Could you check a few things on this drawing? It's one solid part, dimensions in mm from its lowest x, y, z. A direction names the side the tool comes from. Coordinates: 2 decimals unless noted, no trailing zeros. Loops run counter-clockwise (first coordinate to the right, second up) from the corner with the lowest first, then second, coordinate; pieces in that order, holes last. Notation, with made-up numbers: M -37.5,20.25 L -1.5,20.25 A24 ccw -1.5,32.25 Z; hole C 37.5,75 d3. An arc over 180 degrees is marked long. Use one line per item in the form item = value. Start each with the question number.
(1) Imagine slicing it at B-B, the plane y = 25. Please give me the cut outline in (x, z), and give its area (3 significant figures).
(2) Imagine slicing it at A-A, the plane x = 16. Please give me the cut outline in (y, z).
(3) Thinking about a two-plate mould opening in Y: for the marked faces 1, 2 and 3, which applies, +Y half, -Y half, draft (parallel to the pull), parting line (faces both ways), or undercut?
(4) On a 3-axis mill with a long thin cutter (end or side, diameter ignored), from which of +Z, -Z, +X, -X, +Y, -Y can I reach the whole of each face in a straight line? I mean the marked faces 4, 5 and 6. Say none if no direction works.
(5) Will these pins go through, and if not, where does the flat tip stop? P1, Ø6, axis at x = 6.5, z = 7, coming from the +Y side; P2, Ø9, axis at y = 42, z = 33.5, coming from the +X side; P3, Ø4.5, axis at y = 71, z = 19.5, coming from the -X side.
(6) Please list where these lines run through material, in increasing order: L1, parallel to Y at x = 9.5, z = 25; L2, parallel to Y at x = 23, z = 25; L3, parallel to Y at x = 20, z = 14.5.
(7) Imagine slicing it at D-D, the plane x = 8.25. Please give me the cut outline in (y, z), and give its area (3 significant figures).
(8) Imagine slicing it at C-C, the plane z = 25. Please give me the cut outline in (x, y).
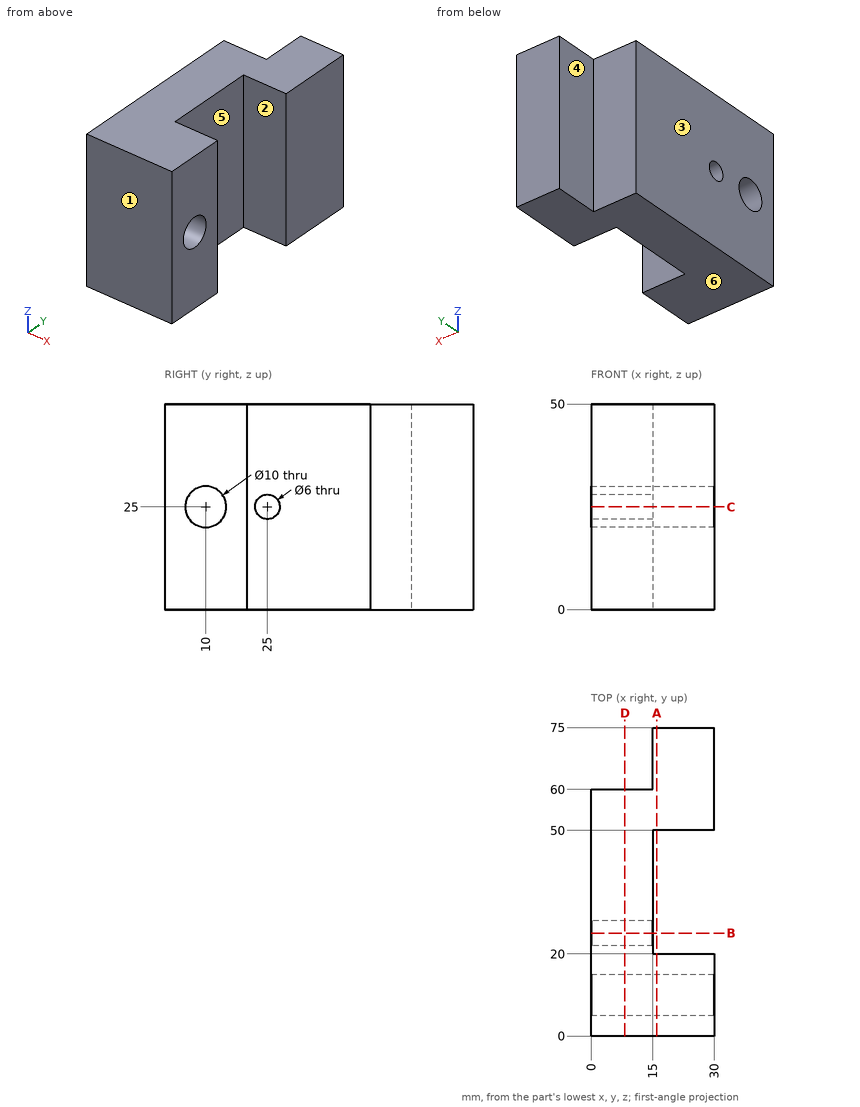
Answer:
q1.outline = M 0,0 L 15,0 L 15,22 L 0,22 Z; M 0,28 L 15,28 L 15,50 L 0,50 Z
q1.area = 660 mm²
q2.outline = M 0,0 L 20,0 L 20,50 L 0,50 Z; M 50,0 L 75,0 L 75,50 L 50,50 Z; hole C 10,25 d10
q3.face_1 = -Y half
q3.face_2 = undercut
q3.face_3 = draft
q4.face_4 = +Z, -Z, -X, +Y
q4.face_5 = +Z, -Z, +X
q4.face_6 = -Z, +X, -X, +Y, -Y
q5.P1 = 60
q5.P2 = 15
q5.P3 = 15
q6.L1 = 0 to 5, 15 to 22, 28 to 60
q6.L2 = 0 to 5, 15 to 20, 50 to 75
q6.L3 = 0 to 20, 50 to 75
q7.outline = M 0,0 L 60,0 L 60,50 L 0,50 Z; hole C 10,25 d10; hole C 25,25 d6
q7.area = 2,890 mm²
q8.outline = M 0,0 L 30,0 L 30,5 L 0,5 Z; M 0,15 L 30,15 L 30,20 L 15,20 L 15,22 L 0,22 Z; M 0,28 L 15,28 L 15,50 L 30,50 L 30,75 L 15,75 L 15,60 L 0,60 Z
